The model under review builds one solid part; all positions refer to its coordinate system, in mm. A direction names the side the tool comes from. Give positions to 0.01 mm unless a question says otherwise; leave off trailing zeros. Order: outer loops, then holes, each group sorted by start corner. A loop starts at its lowest first (then second) coordinate and runs counter-clockwise, first axis right, second up.
```python
from build123d import *

# Parameters (mm, degrees)
SKETCH1_R                = 17.9
BOSS_EXTRUDE1_DEPTH      = 57.5
SKETCH1_3_R              = 5.3
SKETCH1_3_R_2            = 1.5875
BOSS_EXTRUDE2_DEPTH      = 2.8
BOSS_EXTRUDE4_DEPTH      = 57.5
BOSS_EXTRUDE4_DEPTH_BACK = 2
BOSS_EXTRUDE4_START      = -2.8
SKETCH1_5_R              = 1.5875
BOSS_EXTRUDE5_START      = 70.2
SKETCH1_6_R              = 1.5875
BOSS_EXTRUDE5_DEPTH      = 75
SKETCH2_R                = 1.375
CUT_EXTRUDE1_DEPTH       = 3
SKETCH3_W                = 2.8
SKETCH3_H                = 0.5
BOSS_EXTRUDE6_DEPTH      = 7
SKETCH4_R                = 0.625
CUT_EXTRUDE2_DEPTH       = 80.566701578
SKETCH2_3_R              = 6.425
BOSS_EXTRUDE7_DEPTH      = 4.75
BOSS_EXTRUDE8_START      = -38.9
BOSS_EXTRUDE8_DEPTH      = 36
FILLET1_R                = 0.5


with BuildPart() as part:
    # Sketch1 → Boss-Extrude1 (new body)
    with BuildSketch(Plane.XY):
        Circle(SKETCH1_R)
    extrude(amount=BOSS_EXTRUDE1_DEPTH)

    # Sketch1<3> → Boss-Extrude2 (add)
    with BuildSketch(Plane.XY):
        Circle(SKETCH1_3_R)
        Circle(SKETCH1_3_R_2, mode=Mode.SUBTRACT)
    extrude(amount=-BOSS_EXTRUDE2_DEPTH)

    # Sketch1<5> → Boss-Extrude4 (add, two sides: drawn at the far end of the back side and taken through both)
    with BuildSketch(Plane.XY.offset(BOSS_EXTRUDE4_START - BOSS_EXTRUDE4_DEPTH_BACK)):
        Circle(SKETCH1_5_R)
    extrude(amount=BOSS_EXTRUDE4_DEPTH + BOSS_EXTRUDE4_DEPTH_BACK)

    # Sketch1<6> → Boss-Extrude5 (add)
    with BuildSketch(Plane.XY.offset(BOSS_EXTRUDE5_START)):
        Circle(SKETCH1_6_R)
    extrude(amount=-BOSS_EXTRUDE5_DEPTH)

    # Sketch2 → Cut-Extrude1 (cut)
    with BuildSketch(Plane.XY.offset(57.5)):
        with Locations((3.86271243, 11.888206454)):
            Circle(SKETCH2_R)
        with Locations((-3.86271243, -11.888206454)):
            Circle(SKETCH2_R)
    extrude(amount=-CUT_EXTRUDE1_DEPTH, mode=Mode.SUBTRACT)

    # Sketch3 → Boss-Extrude6 (add)
    with BuildSketch(Plane(origin=(0, 0, 0), x_dir=(-1, 0, 0), z_dir=(0, 0, -1))):
        with Locations((0, -14.75)):
            Rectangle(SKETCH3_W, SKETCH3_H)
        with Locations((0, 14.75)):
            Rectangle(SKETCH3_W, SKETCH3_H)
    extrude(amount=BOSS_EXTRUDE6_DEPTH)

    # Sketch4 → Cut-Extrude2 (cut, through all)
    with BuildSketch(Plane(origin=(0, 15, 0), x_dir=(1, 0, 0), z_dir=(0, 1, 0))):
        with Locations(Location((0, 5.5, 0), (0, 0, 270))):
            Circle(SKETCH4_R)
    extrude(amount=-CUT_EXTRUDE2_DEPTH, mode=Mode.SUBTRACT)

    # Sketch2<3> → Boss-Extrude7 (add)
    with BuildSketch(Plane.XY.offset(57.5)):
        Circle(SKETCH2_3_R)
    extrude(amount=BOSS_EXTRUDE7_DEPTH)

    # Sketch5 → Boss-Extrude8 (add)
    with BuildSketch(Plane.XY.offset(57.5).offset(BOSS_EXTRUDE8_START)):
        with BuildLine():
            Line((17.50706481, -3.729970743), (18.093893798, -3.854997695))
            ThreePointArc((18.093893798, -3.854997695), (-17.594545551, 5.716814396), (16.90417837, -7.516565283))
            Line((16.90417837, -7.516565283), (16.355934747, -7.272784787))
            ThreePointArc((16.355934747, -7.272784787), (-17.509729181, 3.717443209), (17.9, 0))
            ThreePointArc((17.9, 0), (17.801495163, -1.875305295), (17.50706481, -3.729970743))
        make_face()
    extrude(amount=BOSS_EXTRUDE8_DEPTH)

    # Fillet1
    fillet1_edges = [part.edges().sort_by_distance(p)[0] for p in [
        (-17.9, 0, 57.5),
        (-5.3, 0, -2.8),
        (-6.425, 0, 57.5),
        (-6.425, 0, 62.25),
    ]]
    fillet(fillet1_edges, radius=FILLET1_R)


solid = part.part
```
1. Take a section at C-C (z = 8.5). Write out the cut boundary in (x, y).
2. Take a section at A-A (z = 29). Write out the cut boundary in (x, y) (3 decimals), and give its area (3 significant figures).
3. To check wall thickness, follow line 1 (Z direction, x = -1.5, y = 15); line 2 (Y direction, x = 11.5, z = 34); line 3 (X direction, y = 10.5, z = 12.5). State the ranges of each line that lie inside material, in increasing order.
4. Take a section at B-B (z = 60). Write out the cut boundary in (x, y) (3 decimals), and give its area (3 significant figures).
5. Draft analysis for pull direction Y (two halves, no side actions). For faces 1 (the flat face through (1.23, -1.23, 62.25)), 2 (the cylindrical face through (-17.336, 6.46, 36.348)), 3 (the cylindrical face through (4.896, -2.03, -1.134)), state which applies: pulls with the +Y half, pulls with the -Y half, needs draft (parallel to the pull), parting line crosses it, or undercut.
6. For faces 4 (the flat face through (0, 15, -3)), 5 (the cylindrical face through (-0.34, -1.55, 66.28)), 6 (the flat face through (0, 0, -4.8)), 7 (the flat face through (2, 0, -2.8)), 8 (the flat face through (0, -15, -3)), list the 3-axis set-ups (+Z, -Z, +X, -X, +Y, -Y) from which the entire face can be reached by the end or side of a thin tool; tool diameter is ignored.
7. Insertion check: pin 1 (4 mm diameter, centred on x = 3, y = -12, fed in from -Z); pin 2 (2 mm diameter, centred on x = 0.5, z = -2, fed in from -Y); pin 3 (2 mm diameter, centred on x = -0.5, z = -2.5, fed in from +Y). Each pin has a flat end and moves straight along its axis. Give the tip position at first contact, or say it passes through.
Answer:
1. outline: circle Ø35.8 at (0, 0)
2. outline: (16.356, -7.273) arc R17.9 ccw to (17.507, -3.73) - (18.094, -3.855) arc R18.5 ccw (long way) to (16.904, -7.517) - close
2. area: 1,070 mm2
3. line 1: z = 0 to 57.5
3. line 2: y = -14.49 to 14.49
3. line 3: x = -14.5 to 14.5
4. outline: circle Ø12.85 at (0, 0)
4. area: 130 mm2
5. face 1: needs draft
5. face 2: parting line crosses it
5. face 3: undercut
6. face 4: -Z, +X, -X, +Y
6. face 5: +Z
6. face 6: -Z, +X, -X
6. face 7: -Z
6. face 8: -Z, +X, -X, -Y
7. pin 1: stops at z = 0
7. pin 2: stops at y = -15
7. pin 3: stops at y = 15
